Part model, mm, in its own coordinate system. A direction names the side the tool comes from. Round coordinates to 2 decimals unless told otherwise and drop trailing zeros. Order: outer loops, then holes, each group sorted by start corner. A loop starts at its lowest first (then second) coordinate and runs counter-clockwise, first axis right, second up. Notation, with made-up numbers: M -20.75,46.25 L 18.25,46.25 A9 ccw 18.25,60.25 Z; hole C 52.5,23 d11. An arc over 180 degrees is marked long. One line per question, with ' | ' between items.
from build123d import *

# Parameters (mm, degrees)
SZKIC1_W                    = 130
SZKIC1_H                    = 60
DODANIE_WYCI_GNI_CIE1_DEPTH = 25
SKORUPA1_T                  = 3
SZKIC3_W                    = 25
SZKIC3_H                    = 60
WYTNIJ_WYCI_GNI_CIE1_DEPTH  = 1.1
DODANIE_WYCI_GNI_CIE2_DEPTH = 3.85
DODANIE_WYCI_GNI_CIE3_DEPTH = 1.6
WYTNIJ_WYCI_GNI_CIE2_DEPTH  = 141.345324112
SZKIC8_R                    = 1.75
DODANIE_WYCI_GNI_CIE4_DEPTH = 25
SZKIC8_2_R                  = 1.75
WYTNIJ_WYCI_GNI_CIE3_DEPTH  = 10
DODANIE_WYCI_GNI_CIE5_START = 5
SZKIC9_R                    = 1.75
DODANIE_WYCI_GNI_CIE5_DEPTH = 5
DODANIE_WYCI_GNI_CIE6_DEPTH = 2
SZKIC11_W                   = 9
SZKIC11_H                   = 9.5
WYTNIJ_WYCI_GNI_CIE4_DEPTH  = 10.5
WYTNIJ_WYCI_GNI_CIE5_REACH  = 144.527
SZKIC15_W                   = 15
SZKIC15_H                   = 12
SZKIC15_H_2                 = 15
SZKIC16_R                   = 3.5
WYTNIJ_WYCI_GNI_CIE6_DEPTH  = 7.35
SZKIC17_R                   = 4.5
SZKIC17_R_2                 = 3.5
SZKIC17_R_3                 = 1.75
DODANIE_WYCI_GNI_CIE7_DEPTH = 14.5


with BuildPart() as part:
    # Szkic1 → Dodanie-wyciągnięcie1 (new body)
    with BuildSketch(Plane.XY):
        Rectangle(SZKIC1_W, SZKIC1_H)
    extrude(amount=DODANIE_WYCI_GNI_CIE1_DEPTH)

    # Skorupa1
    skorupa1_openings = [part.faces().sort_by_distance(p)[0] for p in [
        (0, 0, 25),
    ]]
    offset(amount=SKORUPA1_T, openings=skorupa1_openings, kind=Kind.INTERSECTION)

    # Szkic3 → Wytnij-wyciągnięcie1 (cut)
    with BuildSketch(Plane(origin=(-65, 0, 0), x_dir=(0, 0, -1), z_dir=(1, 0, 0))):
        with Locations((-12.5, 0)):
            Rectangle(SZKIC3_W, SZKIC3_H)
    extrude(amount=-WYTNIJ_WYCI_GNI_CIE1_DEPTH, mode=Mode.SUBTRACT)

    # Szkic4 → Dodanie-wyciągnięcie2 (add)
    with BuildSketch(Plane(origin=(-66.1, 0, 0), x_dir=(0, 0, -1), z_dir=(1, 0, 0))):
        with BuildLine():
            Line((0, 30), (-25, 30))
            Line((-25, 30), (-25, 22.275))
            ThreePointArc((-25, 22.275), (-20.757359313, 20.517640687), (-19, 16.275))
            Line((-19, 16.275), (-19, -16.275))
            ThreePointArc((-19, -16.275), (-20.757359313, -20.517640687), (-25, -22.275))
            Line((-25, -22.275), (-25, -30))
            Line((-25, -30), (0, -30))
            Line((0, -30), (0, 30))
        make_face()
    extrude(amount=DODANIE_WYCI_GNI_CIE2_DEPTH)

    # Szkic5 → Dodanie-wyciągnięcie3 (add)
    with BuildSketch(Plane(origin=(-62.25, 0, 0), x_dir=(0, 0, -1), z_dir=(1, 0, 0))):
        with BuildLine():
            ThreePointArc((-25, 20.775), (-21.818019485, 19.456980515), (-20.5, 16.275))
            Line((-20.5, 16.275), (-20.5, -16.275))
            ThreePointArc((-20.5, -16.275), (-21.818019485, -19.456980515), (-25, -20.775))
            Line((-25, -20.775), (-25, -30))
            Line((-25, -30), (0, -30))
            Line((0, -30), (0, 30))
            Line((0, 30), (-25, 30))
            Line((-25, 30), (-25, 20.775))
        make_face()
    extrude(amount=DODANIE_WYCI_GNI_CIE3_DEPTH)

    # Szkic6 → Wytnij-wyciągnięcie2 (cut, through all)
    with BuildSketch(Plane(origin=(-66.1, 0, 0), x_dir=(0, 0, -1), z_dir=(1, 0, 0))):
        with BuildLine():
            Line((-20.5, -16.275), (-20.5, 16.275))
            ThreePointArc((-20.5, 16.275), (-21.818019485, 19.456980515), (-25, 20.775))
            Line((-25, 20.775), (-25, -20.775))
            ThreePointArc((-25, -20.775), (-21.818019485, -19.456980515), (-20.5, -16.275))
        make_face()
    extrude(amount=-WYTNIJ_WYCI_GNI_CIE2_DEPTH, mode=Mode.SUBTRACT)

    # Szkic8 → Dodanie-wyciągnięcie4 (add)
    # profile 1 of 3: a face of its own
    with BuildSketch(Plane.XY.offset(25)):
        with Locations((-64.325, 27.5875)):
            Circle(SZKIC8_R)
    # profile 2 of 3: a face of its own
    with BuildSketch(Plane.XY.offset(25)):
        with Locations((-64.325, -27.5875)):
            Circle(SZKIC8_R)
    # profile 3 of 3: a face of its own
    with BuildSketch(Plane.XY.offset(25)):
        with BuildLine():
            Line((-19.15, 25), (-19.15, 30))
            Line((-19.15, 30), (-10.15, 30))
            Line((-10.15, 30), (-10.15, 25))
            ThreePointArc((-10.15, 25), (-14.65, 20.5), (-19.15, 25))
        make_face()
        with Locations((-14.65, 25)):
            Circle(SZKIC8_R, mode=Mode.SUBTRACT)
    extrude(amount=-DODANIE_WYCI_GNI_CIE4_DEPTH)

    # Szkic8<2> → Wytnij-wyciągnięcie3 (cut)
    with BuildSketch(Plane.XY.offset(25)):
        with Locations((-64.325, 27.5875)):
            Circle(SZKIC8_2_R)
        with Locations((-64.325, -27.5875)):
            Circle(SZKIC8_2_R)
    extrude(amount=-WYTNIJ_WYCI_GNI_CIE3_DEPTH, mode=Mode.SUBTRACT)

    # Szkic9 → Dodanie-wyciągnięcie5 (add)
    with BuildSketch(Plane.XY.offset(DODANIE_WYCI_GNI_CIE5_START)):
        with Locations((-14.65, 25)):
            Circle(SZKIC9_R)
    extrude(amount=-DODANIE_WYCI_GNI_CIE5_DEPTH)

    # Szkic10 → Dodanie-wyciągnięcie6 (add)
    with BuildSketch(Plane.XY.offset(25)):
        Polygon((-61.65, 31), (-67, 31), (-67, 32), (67, 32), (67, -32), (-67, -32), (-67, -31), (-61.65, -31), (66, -31), (66, 31), (-11.15, 31), (-18.15, 31), align=None)
    extrude(amount=DODANIE_WYCI_GNI_CIE6_DEPTH)

    # Szkic11 → Wytnij-wyciągnięcie4 (cut)
    with BuildSketch(Plane.XY.offset(25)):
        with Locations((-14.65, 25.25)):
            Rectangle(SZKIC11_W, SZKIC11_H)
    extrude(amount=-WYTNIJ_WYCI_GNI_CIE4_DEPTH, mode=Mode.SUBTRACT)

    # Szkic15 → Wytnij-wyciągnięcie5 (cut, up to next)
    with BuildSketch(Plane(origin=(68, 0, 0), x_dir=(0, 0, -1), z_dir=(1, 0, 0)), mode=Mode.PRIVATE) as wytnij_wyci_gni_cie5_sk1:
        with Locations((-24, -14.5)):
            Rectangle(SZKIC15_W, SZKIC15_H)
    wytnij_wyci_gni_cie5_tool1 = extrude(wytnij_wyci_gni_cie5_sk1.sketch, amount=-WYTNIJ_WYCI_GNI_CIE5_REACH, mode=Mode.PRIVATE) & part.part
    # Szkic15 → Wytnij-wyciągnięcie5 (cut, up to next)
    with BuildSketch(Plane(origin=(68, 0, 0), x_dir=(0, 0, -1), z_dir=(1, 0, 0)), mode=Mode.PRIVATE) as wytnij_wyci_gni_cie5_sk2:
        with Locations((-24, 9.5)):
            Rectangle(SZKIC15_W, SZKIC15_H_2)
    wytnij_wyci_gni_cie5_tool2 = extrude(wytnij_wyci_gni_cie5_sk2.sketch, amount=-WYTNIJ_WYCI_GNI_CIE5_REACH, mode=Mode.PRIVATE) & part.part
    add(wytnij_wyci_gni_cie5_tool1.solids().sort_by_distance((68, -14.5, 24))[0], mode=Mode.SUBTRACT)
    add(wytnij_wyci_gni_cie5_tool2.solids().sort_by_distance((68, 9.5, 24))[0], mode=Mode.SUBTRACT)

    # Szkic16 → Wytnij-wyciągnięcie6 (cut)
    with BuildSketch(Plane.ZY.offset(68)):
        with Locations((5, 25)):
            Circle(SZKIC16_R)
    extrude(amount=-WYTNIJ_WYCI_GNI_CIE6_DEPTH, mode=Mode.SUBTRACT)

    # Szkic17 → Dodanie-wyciągnięcie7 (add)
    # profile 1 of 2: a face of its own
    with BuildSketch(Plane.XY):
        with Locations((50, -15)):
            Circle(SZKIC17_R)
        with Locations((50, -15)):
            Circle(SZKIC17_R_2, mode=Mode.SUBTRACT)
    # profile 2 of 2: a face of its own
    with BuildSketch(Plane.XY):
        with BuildLine():
            Line((52, 27), (52, 30))
            Line((52, 30), (58, 30))
            Line((58, 30), (58, 27))
            ThreePointArc((58, 27), (55, 24), (52, 27))
        make_face()
        with Locations((55, 27)):
            Circle(SZKIC17_R_3, mode=Mode.SUBTRACT)
    extrude(amount=DODANIE_WYCI_GNI_CIE7_DEPTH)


solid = part.part
1) Two-plate mould, pull along Z, no slides. Class faces 4 (the face through (55, 27, 0)), 5 (the face through (-19.15, 27, 7)), 6 (the face through (-64.38, 28.47, 4.54)): released by +Z, released by -Z, zero draft, split by the parting line, or undercut.
The answers:
face 4: released by +Z | face 5: zero draft | face 6: undercut
2) Saw through at C-C (x = -14.65). List the corners of the cut face in (y, z), plus the area to 4 significant figures.
The answers:
outline: M -33,-3 L 33,-3 L 33,25 L 32,25 L 32,27 L 31,27 L 31,25 L 30,25 L 30,14.5 L 26.75,14.5 L 26.75,5 L 23.25,5 L 23.25,14.5 L 20.5,14.5 L 20.5,0 L -30,0 L -30,25 L -31,25 L -31,27 L -32,27 L -32,25 L -33,25 Z | area: 456.5 mm²
3) Saw through at D-D (x = 50). List the corners of the cut face in (y, z).
The answers:
outline: M -33,-3 L 33,-3 L 33,25 L 32,25 L 32,27 L 31,27 L 31,25 L 30,25 L 30,0 L -10.5,0 L -10.5,14.5 L -11.5,14.5 L -11.5,0 L -18.5,0 L -18.5,14.5 L -19.5,14.5 L -19.5,0 L -30,0 L -30,25 L -31,25 L -31,27 L -32,27 L -32,25 L -33,25 Z
4) Probe line 1 (Y direction, x = 50, z = 10.25); line 2 (Y direction, x = -3, z = 23.75); line 3 (Y direction, x = 55, z = 10.5). List the from-to ranges inside material, lowest first. Write a range as [from, to].
The answers:
line 1: y = [-33, -30], [-19.5, -18.5], [-11.5, -10.5], [30, 33] | line 2: y = [-33, -30], [30, 33] | line 3: y = [-33, -30], [24, 25.25], [28.75, 33]
5) Which spindle directions (+Z, -Z, +X, -X, +Y, -Y) get a long thin tool onto all of the face, cutting with end or side? Do faces 1 (the face through (-68, 0, 11)), 2 (the face through (67, 2, 21)), 3 (the face through (58, 29, 7)). Say none if no direction does.
The answers:
face 1: +Z, -Z, -X, +Y, -Y | face 2: +Z, +X | face 3: +Z
6) Saw through at B-B (x = 6). List the corners of the cut face in (y, z).
The answers:
outline: M -33,-3 L 33,-3 L 33,25 L 32,25 L 32,27 L 31,27 L 31,25 L 30,25 L 30,0 L -30,0 L -30,25 L -31,25 L -31,27 L -32,27 L -32,25 L -33,25 Z
7) Drop flat-ended pins along their axis: pin 1 (3 mm diameter, centred on x = -30, y = 19, fed in from +Z); pin 2 (0.8 mm diameter, centred on y = 31.5, z = 25.5, fed in from -X); pin 3 (2.5 mm diameter, centred on x = -15.5, y = 23.5, fed in from +Z). Give the stop position or say it passes through.
The answers:
pin 1: stops at z = 0 | pin 2: stops at x = -67 | pin 3: stops at z = 14.5
8) Saw through at A-A (z = 6.25). List the corners of the cut face in (x, y), plus the area to 3 significant figures.
The answers:
outline: M -68,-33 L 68,-33 L 68,33 L -68,33 L -68,28.27 L -60.65,28.27 L -60.65,30 L -19.15,30 L -19.15,25 A4.5 ccw -10.15,25 L -10.15,30 L 52,30 L 52,27 A3 ccw 58,27 L 58,30 L 65,30 L 65,-30 L -60.65,-30 L -60.65,21.73 L -68,21.73 Z; C 50,-15 d9; hole C -14.65,25 d3.5; hole C 50,-15 d7; hole C 55,27 d3.5 | area: 1,500 mm²
